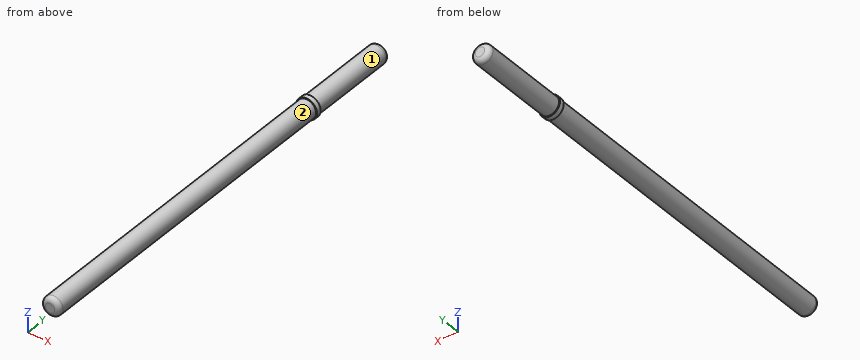
```python
from build123d import *

# Parameters (mm, degrees)
SKETCH_1_R        = 0.98
EXTRUDE_1_DEPTH   = 45
FILLET_1_R        = 0.5
SKETCH_2_R        = 1.08
SKETCH_2_R_2      = 0.98
EXTRUDE_1_2_DEPTH = 0.5


with BuildPart() as part:
    # 草图1 → Extrude 1 (new body)
    with BuildSketch(Plane(origin=(0, 0, 0), x_dir=(1, 0, 0), z_dir=(0, 1, 0))):
        Circle(SKETCH_1_R)
    extrude(amount=EXTRUDE_1_DEPTH)

    # 圆角1
    fillet_1_edges = [part.edges().sort_by_distance(p)[0] for p in [
        (-0.98, 0, 0),
        (-0.98, 45, 0),
    ]]
    fillet(fillet_1_edges, radius=FILLET_1_R)

    # 草图2 → Extrude 1 2 (add)
    with BuildSketch(Plane(origin=(0, 35.5, 0), x_dir=(1, 0, 0), z_dir=(0, 1, 0))):
        Circle(SKETCH_2_R)
        Circle(SKETCH_2_R_2, mode=Mode.SUBTRACT)
    extrude(amount=-EXTRUDE_1_2_DEPTH)


solid = part.part
```
Geometry check sheet. Reference: the model listing, model coordinates, mm. Face numbers are marked on the shaded views. A direction names the side the tool comes from. Coordinates: 2 decimals unless noted, no trailing zeros. Loops run counter-clockwise (first coordinate to the right, second up) from the corner with the lowest first, then second, coordinate; pieces in that order, holes last.
Item 1: Access from +Z, -Z, +X, -X, +Y, -Y to the whole of each face (thin tool, end or side, straight path). Record for the marked faces 1 and 2.
Item 2: Thickness scan on line 1 (Z direction, x = 0.05, y = 42.5); line 2 (Y direction, x = 1, z = -0.3); line 3 (X direction, y = 40.5, z = 0.1). Record the ranges inside material, lowest first.
Item 3: Sectioned sample at A-A, the plane y = 41. Record the boundary of the cut face in (x, z), then the cut area to 3 significant figures.
Check result:
1. face 1: +Y
1. face 2: -Y
2. line 1: z = -0.98 to 0.98
2. line 2: y = 35 to 35.5
2. line 3: x = -0.97 to 0.97
3. outline: circle Ø1.96 at (0, 0)
3. area: 3.02 mm2
